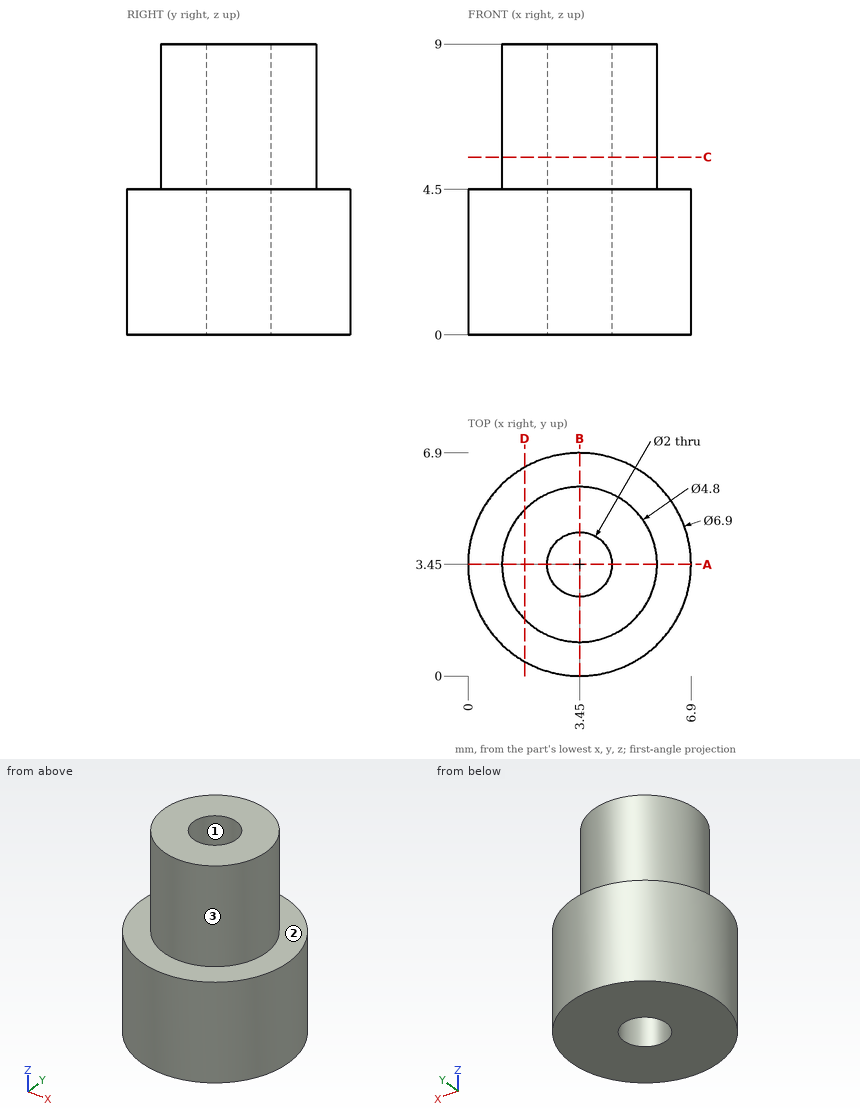
Design review of the part shown in the three views and the two pictorial views. Dimensions are in mm from the part's minimum x, y and z. Give positions to 0.01 mm unless a question says otherwise; leave off trailing zeros. Write each loop counter-clockwise with the first axis right and the second up, starting at its lowest first coordinate (ties: lowest second). Pieces come first, ordered by that corner, then holes. Notation, with made-up numbers: (13.5, 11) -> (26.5, 11) arc R16 ccw to (26.5, 34) -> close; hole circle Ø11 at (83, -19.75). An arc over 180 degrees is marked (long way). Answer in a Markdown table with one row per item.
1) Add section A-A on y = 3.45. State the section outline as (x, z) points, plus the area to 4 significant figures.
Worked answers:
| item | result |
|---|---|
| outline | (0, 0) -> (2.45, 0) -> (2.45, 9) -> (1.05, 9) -> (1.05, 4.5) -> (0, 4.5) -> close; (4.45, 0) -> (6.9, 0) -> (6.9, 4.5) -> (5.85, 4.5) -> (5.85, 9) -> (4.45, 9) -> close |
| area | 34.65 mm² |
2) Mouldability with a two-part tool opening along Y and no side actions: class the marked faces 1, 2 and 3 as +Y half, -Y half, draft (parallel to the pull), parting line (faces both ways), or undercut.
Worked answers:
| item | result |
|---|---|
| face 1 | undercut |
| face 2 | draft |
| face 3 | parting line |
3) Clearance check with flat-ended pins moving along their axes: P1, Ø3, axis at x = 1.5, z = 7, coming from the -Y side; P2, Ø1, axis at x = 6, y = 2, coming from the +Z side; P3, Ø4, axis at x = 5.5, z = 6, coming from the +Y side. State where each tip first meets the part, or that it passes through.
Worked answers:
| item | result |
|---|---|
| P1 | y = 1.09 |
| P2 | z = 4.5 |
| P3 | y = 6.82 |
4) Add section D-D on x = 1.75. State the section outline as (y, z) points, plus the area to 3 significant figures.
Worked answers:
| item | result |
|---|---|
| outline | (0.45, 0) -> (6.45, 0) -> (6.45, 4.5) -> (5.14, 4.5) -> (5.14, 9) -> (1.76, 9) -> (1.76, 4.5) -> (0.45, 4.5) -> close |
| area | 42.3 mm² |
5) For L1, parallel to Y at x = 3.45, z = 5; L2, parallel to Z at x = 5, y = 0.5; L3, parallel to Y at x = 3, z = 1.75, list the stretches that pass through material, from the lowest coordinate up. Write a range as [from, to].
Worked answers:
| item | result |
|---|---|
| L1 | [1.05, 2.45], [4.45, 5.85] |
| L2 | [0, 4.5] |
| L3 | [0.03, 2.56], [4.34, 6.87] |
6) Add section C-C on z = 5.5. State the section outline as (x, y) points.
Worked answers:
| item | result |
|---|---|
| outline | circle Ø4.8 at (3.45, 3.45); hole circle Ø2 at (3.45, 3.45) |
